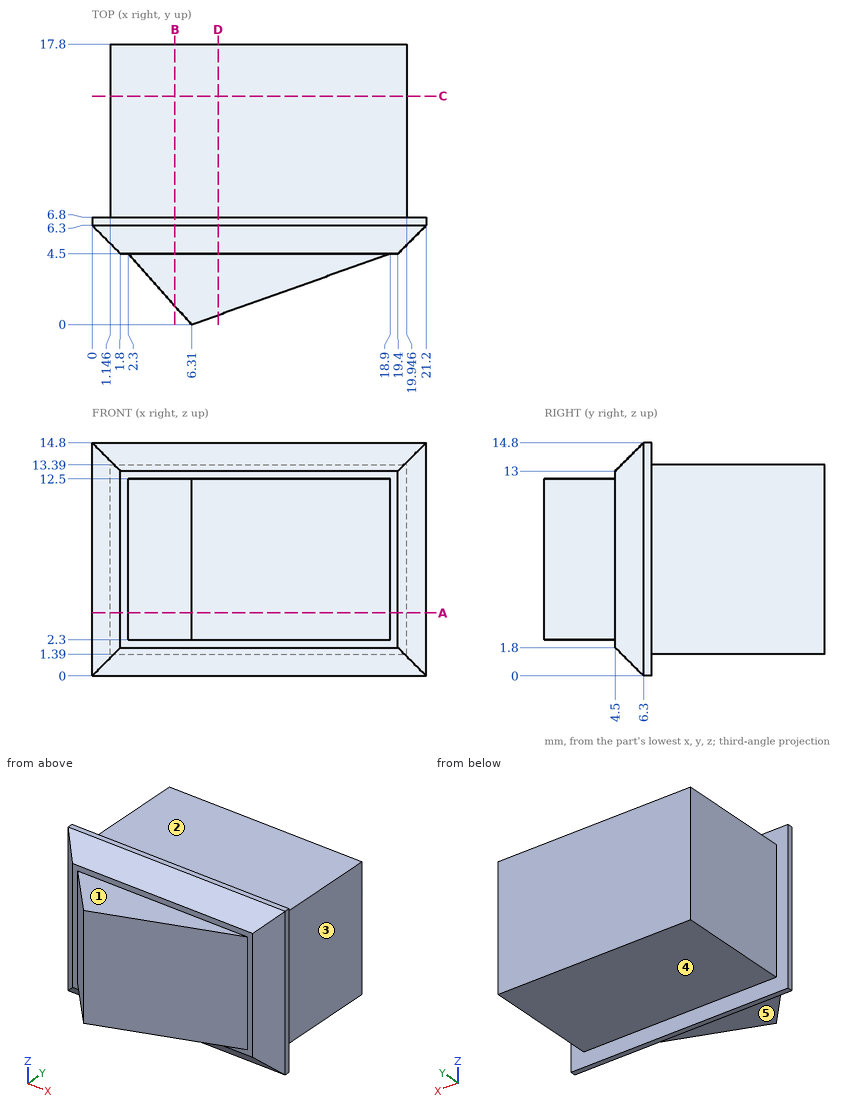
Drawing for the job (mm, zero at the part's lowest x, y, z). A direction names the side the tool comes from. Round coordinates to 2 decimals unless told otherwise and drop trailing zeros. Write each loop counter-clockwise with the first axis right and the second up, starting at its lowest first coordinate (ties: lowest second). Pieces come first, ordered by that corner, then holes.
Item 1: Band-saw the part on D-D on x = 8. Write the cut outline in (y, z).
Filled in:
outline: (0.6, 2.3) - (4.5, 2.3) - (4.5, 1.8) - (6.3, 0) - (6.8, 0) - (6.8, 1.39) - (17.8, 1.39) - (17.8, 13.39) - (6.8, 13.39) - (6.8, 14.8) - (6.3, 14.8) - (4.5, 13) - (4.5, 12.5) - (0.6, 12.5) - close
Item 2: Band-saw the part on C-C on y = 14.5. Write the cut outline in (x, z).
Filled in:
outline: (1.15, 1.39) - (19.95, 1.39) - (19.95, 13.39) - (1.15, 13.39) - close
Item 3: Tool access for the marked faces 1, 2, 3, 4 and 5: list every direction of +Z, -Z, +X, -X, +Y, -Y with a clear straight run to the whole face (end or side of a thin tool).
Filled in:
face 1: +Z, +X, -X, -Y
face 2: +Z, +X, -X, +Y
face 3: +Z, -Z, +X, +Y
face 4: -Z, +X, -X, +Y
face 5: -Z, +X, -X, -Y
Item 4: Band-saw the part on B-B on x = 5.25. Write the cut outline in (y, z), then the cut area to 3 significant figures.
Filled in:
outline: (1.19, 2.3) - (4.5, 2.3) - (4.5, 1.8) - (6.3, 0) - (6.8, 0) - (6.8, 1.39) - (17.8, 1.39) - (17.8, 13.39) - (6.8, 13.39) - (6.8, 14.8) - (6.3, 14.8) - (4.5, 13) - (4.5, 12.5) - (1.19, 12.5) - close
area: 197 mm2
Item 5: Band-saw the part on A-A on z = 4. Write the cut outline in (x, y).
Filled in:
outline: (0, 6.3) - (1.8, 4.5) - (2.3, 4.5) - (6.31, 0) - (18.9, 4.5) - (19.4, 4.5) - (21.2, 6.3) - (21.2, 6.8) - (19.95, 6.8) - (19.95, 17.8) - (1.15, 17.8) - (1.15, 6.8) - (0, 6.8) - close
Item 6: Drop flat-ended pins along their axis: pin 1 Ø6 at (x, y) = (11.5, 3.5) entering from +Z; pin 2 Ø5 at (y, z) = (10.5, 12.5) entering from -X; pin 3 Ø5.5 at (y, z) = (14.5, 10) entering from +X; pin 4 Ø2 at (x, y) = (12, 2) entering from -Z. Give the stop position or say it passes through.
Filled in:
pin 1: stops at z = 14.8
pin 2: stops at x = 1.15
pin 3: stops at x = 19.95
pin 4: stops at z = 2.3
Item 7: Drill centre lines: L1, parallel to X at y = 15.5, z = 7.75; L2, parallel to Z at x = 17.25, y = 14.75; L3, parallel to Z at x = 11.25, y = 2.25. Where is each one in solid material? Low to high.
Filled in:
L1: x = 1.15 to 19.95
L2: z = 1.39 to 13.39
L3: z = 2.3 to 12.5
